Verification items for the finished model (mm, model axes). A direction names the side the tool comes from. Round coordinates to 2 decimals unless told otherwise and drop trailing zeros. Write each loop counter-clockwise with the first axis right and the second up, starting at its lowest first coordinate (ties: lowest second). Pieces come first, ordered by that corner, then holes. Notation, with made-up numbers: M 65,-33.5 L 122,-33.5 A7 cw 122,-27.5 Z; hole C 41,62.5 d9. An arc over 180 degrees is marked long. One line per item, written item: value. Start each with the question number.
from build123d import *

# Parameters (mm, degrees)
SKETCH1_W                = 50
SKETCH1_H                = 60
BOSS_EXTRUDE1_DEPTH      = 25
CUT_EXTRUDE1_START       = -16.25
SKETCH2_R                = 21
CUT_EXTRUDE1_DEPTH       = 17.5
CUT_EXTRUDE2_START       = -12
SKETCH3_R                = 7.6
CUT_EXTRUDE2_DEPTH       = 26
SKETCH4_R                = 5
CUT_EXTRUDE3_DEPTH       = 4
SKETCH5_R                = 1.75
CUT_EXTRUDE4_DEPTH       = 10
CHAMFER1_SIZE            = 5
SKETCH6_R                = 2
CUT_EXTRUDE5_DEPTH       = 10
SKETCH7_W                = 11
SKETCH7_H                = 5.906734889
CUT_EXTRUDE6_DEPTH       = 9
CHAMFER2_SIZE            = 5
CHAMFER2_OF_MIRROR1_SIZE = 5
CHAMFER3_SIZE            = 3
CUT_EXTRUDE8_START       = 25
SKETCH10_R               = 2
CUT_EXTRUDE8_DEPTH       = 25.371044145
CUT_EXTRUDE10_DEPTH      = 64.442887702
CUT_EXTRUDE10_DEPTH_BACK = 64.442887702
SKETCH12_R               = 6
FILLET1_R                = 8
SKETCH16_R               = 7.75
CUT_EXTRUDE13_DEPTH      = 8
SKETCH17_W               = 20
SKETCH17_H               = 10
BOSS_EXTRUDE2_DEPTH      = 5
SKETCH18_R               = 3.25
CUT_EXTRUDE14_DEPTH      = 10
SKETCH19_R               = 5
CUT_EXTRUDE15_DEPTH      = 4
FILLET2_R                = 5


with BuildPart() as part:
    # Sketch1 → Boss-Extrude1 (new body)
    with BuildSketch(Plane(origin=(0, 0, 0), x_dir=(1, 0, 0), z_dir=(0, 1, 0))):
        Rectangle(SKETCH1_W, SKETCH1_H)
    extrude(amount=BOSS_EXTRUDE1_DEPTH)

    # Sketch2 → Cut-Extrude1 (cut)
    with BuildSketch(Plane.ZY.offset(25).offset(CUT_EXTRUDE1_START)):
        with Locations((0, 25)):
            Circle(SKETCH2_R)
    extrude(amount=-CUT_EXTRUDE1_DEPTH, mode=Mode.SUBTRACT)

    # Sketch3 → Cut-Extrude2 (cut)
    with BuildSketch(Plane.ZY.offset(25).offset(CUT_EXTRUDE2_START)):
        with Locations((0, 25)):
            Circle(SKETCH3_R)
    extrude(amount=-CUT_EXTRUDE2_DEPTH, mode=Mode.SUBTRACT)

    # Sketch4 → Cut-Extrude3 (cut)
    with BuildSketch(Plane.XY.offset(30)):
        with Locations((0, 25)):
            Circle(SKETCH4_R)
    extrude(amount=-CUT_EXTRUDE3_DEPTH, mode=Mode.SUBTRACT)

    # Sketch5 → Cut-Extrude4 (cut)
    with BuildSketch(Plane.XZ):
        with Locations(Location((-10, 20, 0), (0, 0, 270))):
            Circle(SKETCH5_R)
        with Locations(Location((10, 20, 0), (0, 0, 270))):
            Circle(SKETCH5_R)
        with Locations(Location((-10, -20, 0), (0, 0, 270))):
            Circle(SKETCH5_R)
        with Locations(Location((10, -20, 0), (0, 0, 270))):
            Circle(SKETCH5_R)
    extrude(amount=-CUT_EXTRUDE4_DEPTH, mode=Mode.SUBTRACT)

    # Chamfer1
    chamfer1_edges = [part.edges().sort_by_distance(p)[0] for p in [
        (0, 0, -30),
    ]]
    chamfer(chamfer1_edges, length=CHAMFER1_SIZE)

    # Sketch6 → Cut-Extrude5 (cut)
    with BuildSketch(Plane(origin=(0, 0, -30), x_dir=(-1, 0, 0), z_dir=(0, 0, -1))):
        with Locations((-20, 15)):
            Circle(SKETCH6_R)
        with Locations((20, 15)):
            Circle(SKETCH6_R)
    extrude(amount=-CUT_EXTRUDE5_DEPTH, mode=Mode.SUBTRACT)

    # Sketch7 → Cut-Extrude6 (cut)
    with BuildSketch(Plane(origin=(25, 0, 0), x_dir=(0, 0, -1), z_dir=(1, 0, 0))):
        with Locations((-10, 2.953367444)):
            Rectangle(SKETCH7_W, SKETCH7_H)
        with Locations((10, 2.953367444)):
            Rectangle(SKETCH7_W, SKETCH7_H)
    cut_extrude6 = extrude(amount=-CUT_EXTRUDE6_DEPTH, mode=Mode.SUBTRACT)

    # Chamfer2
    chamfer2_edges = [part.edges().sort_by_distance(p)[0] for p in [
        (16, 5.906734889, 10),
        (16, 5.906734889, -10),
    ]]
    chamfer(chamfer2_edges, length=CHAMFER2_SIZE)

    # Mirror1: Cut-Extrude6 across plane
    add(cut_extrude6.mirror(Plane(origin=(0, 0, 0), x_dir=(0, 0, 1), z_dir=(1, 0, 0))), mode=Mode.SUBTRACT)

    # Chamfer2 of Mirror1
    chamfer2_of_mirror1_edges = [part.edges().sort_by_distance(p)[0] for p in [
        (-16, 5.906734889, 10),
        (-16, 5.906734889, -10),
    ]]
    chamfer(chamfer2_of_mirror1_edges, length=CHAMFER2_OF_MIRROR1_SIZE)

    # Chamfer3
    chamfer3_edges = [part.edges().sort_by_distance(p)[0] for p in [
        (-25, 15, -30),
        (25, 15, -30),
    ]]
    chamfer(chamfer3_edges, length=CHAMFER3_SIZE - 0.0001)  # a hair under: the kernel refuses the full size

    # Sketch10 → Cut-Extrude8 (cut, through all)
    with BuildSketch(Plane(origin=(0, -2.5, -2.5), x_dir=(1, 0, 0), z_dir=(0, 0.7071067811865475, 0.7071067811865477)).offset(CUT_EXTRUDE8_START)):
        with Locations(Location((-20, 1.464466094, 0), (0, 0, 90))):
            Circle(SKETCH10_R)
        with Locations(Location((20, 1.464466094, 0), (0, 0, 90))):
            Circle(SKETCH10_R)
    cut_extrude8 = extrude(amount=CUT_EXTRUDE8_DEPTH, mode=Mode.SUBTRACT)

    # Mirror2: Cut-Extrude8 across plane
    add(cut_extrude8.mirror(Plane.XY), mode=Mode.SUBTRACT)

    # Sketch12 → Cut-Extrude10 (cut, two sides: drawn at the far end of the back side and taken through both)
    with BuildSketch(Plane.ZY.offset(25).offset(-CUT_EXTRUDE10_DEPTH_BACK)):
        with Locations((0, 25)):
            Circle(SKETCH12_R)
    extrude(amount=CUT_EXTRUDE10_DEPTH + CUT_EXTRUDE10_DEPTH_BACK, mode=Mode.SUBTRACT)

    # Fillet1
    fillet1_edges = [part.edges().sort_by_distance(p)[0] for p in [
        (25, 19, 0),
        (-25, 19, 0),
    ]]
    fillet(fillet1_edges, radius=FILLET1_R)

    # Sketch16 → Cut-Extrude13 (cut)
    with BuildSketch(Plane.XY.offset(26)):
        with Locations((0, 25)):
            Circle(SKETCH16_R)
    extrude(amount=-CUT_EXTRUDE13_DEPTH, mode=Mode.SUBTRACT)

    # Sketch17 → Boss-Extrude2 (add)
    with BuildSketch(Plane.XY.offset(30)):
        with Locations((0, 20)):
            Rectangle(SKETCH17_W, SKETCH17_H)
    extrude(amount=BOSS_EXTRUDE2_DEPTH)

    # Sketch18 → Cut-Extrude14 (cut)
    with BuildSketch(Plane(origin=(0, 0, 30), x_dir=(-1, 0, 0), z_dir=(0, 0, -1))):
        with Locations((0, 25)):
            Circle(SKETCH18_R)
    extrude(amount=-CUT_EXTRUDE14_DEPTH, mode=Mode.SUBTRACT)

    # Sketch19 → Cut-Extrude15 (cut)
    with BuildSketch(Plane.XY.offset(35)):
        with Locations((0, 25)):
            Circle(SKETCH19_R)
    extrude(amount=-CUT_EXTRUDE15_DEPTH, mode=Mode.SUBTRACT)

    # Fillet2
    fillet2_edges = [part.edges().sort_by_distance(p)[0] for p in [
        (-10, 20, 30),
        (0, 15, 30),
        (10, 20, 30),
    ]]
    fillet(fillet2_edges, radius=FILLET2_R - 0.0001)  # a hair under: the kernel refuses the full size


solid = part.part
1) Access from +Z, -Z, +X, -X, +Y, -Y to the whole of each face (thin tool, end or side, straight path). Record for faces 1 (the flat face through (-22, 2, 4.5)), 2 (the flat face through (10, 10, -20)), 3 (the flat face through (0, 19, 26)), 4 (the cylindrical face through (0, 20, 33)).
2) Cross-section at D-D (y = 23.25). State how many separate pieces and enclosed holes the cut face has, then the cut area to 3 significant figures.
3) Mould release check, pull along X, two halves, no side actions. Record for faces 5 (the flat face through (-23, 13, -29)), 6 (the cylindrical face through (-20, 17, -25)), 7 (the flat face through (-0.3, 9.5, 30)): pulls with the +X half, pulls with the -X half, needs draft (parallel to the pull), parting line crosses it, or undercut.
4) Thickness scan on line 1 (X direction, y = 6.5, z = 4); line 2 (X direction, y = 7, z = 20); line 3 (Y direction, x = 20, z = -27). Record the ranges inside material, lowest first.
5) Cross-section at B-B (z = 0). Record the boundary of the cut face in (x, y).
6) Cross-section at C-C (y = 8). Record the boundary of the cut face in (x, z), then the cut area to 3 significant figures.
7) Gauge pin test, flat ends, axial feed: pin 1 Ø3 at (x, y) = (21.5, 2) entering from -Z; pin 2 Ø4.5 at (x, y) = (20.5, 2.5) entering from +Z; pin 3 Ø1.8 at (x, y) = (-21.5, 2.5) entering from -Z. Record the tip position at first contact, or that the pin passes through.
Results below:
1. face 1: -X, -Y
1. face 2: -Y
1. face 3: +Y
1. face 4: +Z, +Y
2. separate pieces: 3
2. enclosed holes: 4
2. area: 1,680 mm²
3. face 5: pulls with the -X half
3. face 6: undercut
3. face 7: needs draft
4. line 1: x = -25 to -8.75, 8.75 to 25
4. line 2: x = -25 to -11.75, -8.25 to 8.25, 11.75 to 25
4. line 3: y = 2 to 13, 17 to 25
5. outline: M -25,0 L 25,0 L 25,11 A8 ccw 17,19 L 13,19 L 13,17.4 L 8.75,17.4 L 8.75,4 L -8.75,4 L -8.75,17.4 L -13,17.4 L -13,19 L -17,19 A8 ccw -25,11 Z
6. outline: M -25,-27 L -22,-30 L 22,-30 L 25,-27 L 25,30 L -25,30 Z; hole C -10,-20 d3.5; hole C -10,20 d3.5; hole M -8.75,-12.33 L 8.75,-12.33 L 8.75,12.33 L -8.75,12.33 Z; hole C 10,-20 d3.5; hole C 10,20 d3.5
6. area: 2,520 mm²
7. pin 1: stops at z = -28.5
7. pin 2: stops at z = 30
7. pin 3: stops at z = -28.4
